Geometry: see drawing. Coordinates: mm, zero at the bounding-box minimum. A direction names the side the tool comes from. Give positions to 0.01 mm unless a question says otherwise; leave off trailing zeros. Loops run counter-clockwise (first coordinate to the right, second up) from the corner with the lowest first, then second, coordinate; pieces in that order, holes last. Notation, with made-up numbers: M 74.25,44.25 L 114.25,44.25 A9 cw 114.25,58.25 Z; hole C 52.25,1.5 d10. An arc over 180 degrees is marked long. Put each result on its own line as item: value.
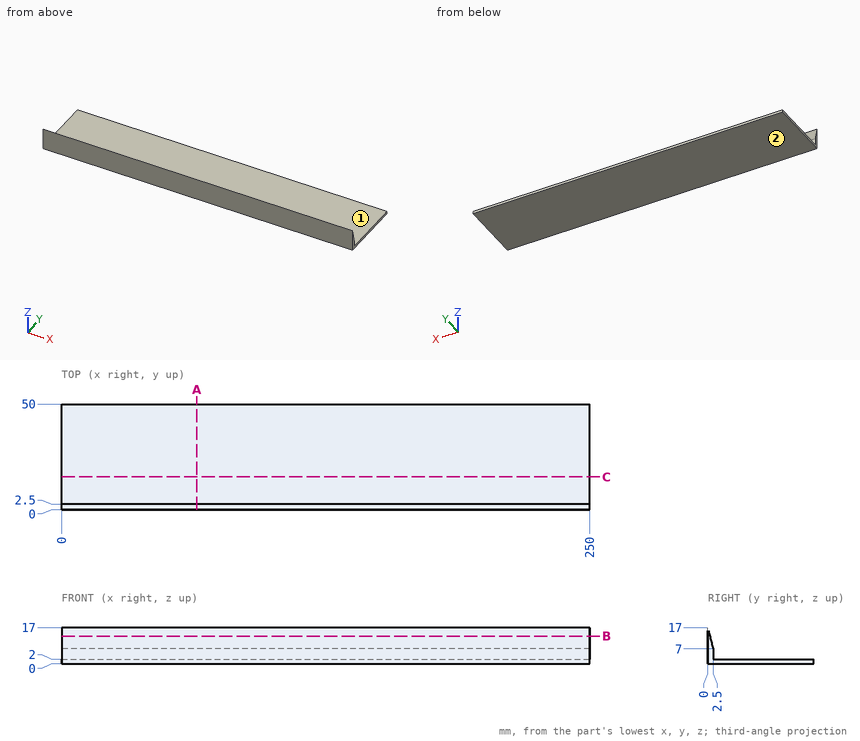
Item 1: Pin query (flat end, axial travel): pin 1 Ø2.5 at (x, z) = (116, 4.5) entering from +Y; pin 2 Ø1 at (x, z) = (134.5, 11.5) entering from +Y; pin 3 Ø12 at (x, y) = (113, 12) entering from -Z; pin 4 Ø2 at (x, y) = (89.5, 23.5) entering from +Z. Return the tip coordinate at first contact, or that it passes through.
Output values:
pin 1: y = 2.5
pin 2: y = 1.5
pin 3: z = 0
pin 4: z = 2
Item 2: Section C-C on y = 15.5. Output: boundary loops of the cut face in (x, z), then the cut area to 3 significant figures.
Output values:
outline: M 0,0 L 250,0 L 250,2 L 0,2 Z
area: 500 mm²
Item 3: Section A-A on x = 64. Output: boundary loops of the cut face in (y, z).
Output values:
outline: M 0,0 L 50,0 L 50,2 L 2.5,2 L 2.5,7 L 0,17 Z
Item 4: Set-up query: the marked faces 1 and 2. Return all of +Z, -Z, +X, -X, +Y, -Y with unobstructed straight access to the full face (end or side cutting, diameter ignored); none if empty.
Output values:
face 1: +Z, +X, -X, +Y
face 2: -Z, +X, -X, +Y, -Y
Item 5: Line query: probe 1 along Z at (x, y) = (21, 36.5); probe 2 along Y at (x, z) = (155.5, 3); probe 3 along Y at (x, z) = (177, 10). Output: solid intervals per line, ascending. Write a range as [from, to].
Output values:
probe 1: [0, 2]
probe 2: [0, 2.5]
probe 3: [0, 1.75]
Item 6: Section B-B on z = 13. Output: boundary loops of the cut face in (x, y), then the cut area to 3 significant figures.
Output values:
outline: M 0,0 L 250,0 L 250,1 L 0,1 Z
area: 250 mm²
